Model file for the job. Use its own axes, mm. Face numbers are marked on the shaded views. A direction names the side the tool comes from. Give positions to 0.01 mm unless a question says otherwise; leave off trailing zeros. Order: outer loops, then holes, each group sorted by start corner. A loop starts at its lowest first (then second) coordinate and runs counter-clockwise, first axis right, second up. Notation, with made-up numbers: (-29, 28) -> (-23, 28) arc R28 cw to (-23, 58) -> close; hole circle Ø1 at (-37, 20.5). An arc over 180 degrees is marked (long way). Answer in a Markdown table with one row per item. Add a question column.
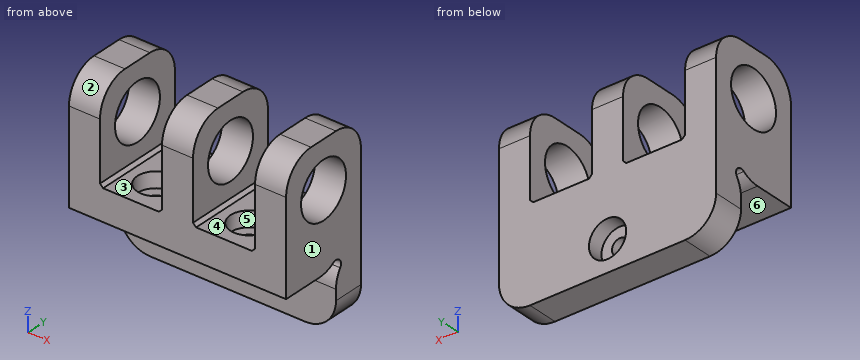
from build123d import *

# Parameters (mm, degrees)
SZKIC1_W                    = 70
SZKIC1_H                    = 30
DODANIE_WYCI_GNI_CIE1_DEPTH = 10
SZKIC2_W                    = 70
SZKIC2_H                    = 10
DODANIE_WYCI_GNI_CIE2_DEPTH = 20
SZKIC3_R                    = 2
WYTNIJ_WYCI_GNI_CIE1_DEPTH  = 75.330343737
ZAOKR_GLENIE1_R             = 10
SZKIC4_W                    = 10
SZKIC4_H                    = 30
DODANIE_WYCI_GNI_CIE3_DEPTH = 30
SZKIC5_R                    = 2.6
WYTNIJ_WYCI_GNI_CIE2_DEPTH  = 49.476798574
SZKIC6_R                    = 6
WYTNIJ_WYCI_GNI_CIE3_DEPTH  = 5
SZKIC7_R                    = 2.6
WYTNIJ_WYCI_GNI_CIE4_DEPTH  = 62.032778079
SZKIC8_R                    = 6
WYTNIJ_WYCI_GNI_CIE5_DEPTH  = 5
ZAOKR_GLENIE2_R             = 10
SZKIC9_R                    = 9
WYTNIJ_WYCI_GNI_CIE6_DEPTH  = 83.006097334
SFAZOWANIE1_SIZE            = 1


with BuildPart() as part:
    # Szkic1 → Dodanie-wyciągnięcie1 (new body)
    with BuildSketch(Plane.XY):
        Rectangle(SZKIC1_W, SZKIC1_H)
    extrude(amount=DODANIE_WYCI_GNI_CIE1_DEPTH)

    # Szkic2 → Dodanie-wyciągnięcie2 (add)
    with BuildSketch(Plane(origin=(0, 0, 0), x_dir=(-1, 0, 0), z_dir=(0, 0, -1))):
        with Locations((0, 10)):
            Rectangle(SZKIC2_W, SZKIC2_H)
    extrude(amount=DODANIE_WYCI_GNI_CIE2_DEPTH)

    # Szkic3 → Wytnij-wyciągnięcie1 (cut, through all)
    with BuildSketch(Plane(origin=(35, 0, 0), x_dir=(0, 0, -1), z_dir=(1, 0, 0))):
        with Locations((0, 5)):
            Circle(SZKIC3_R)
    extrude(amount=-WYTNIJ_WYCI_GNI_CIE1_DEPTH, mode=Mode.SUBTRACT)

    # Zaokrąglenie1
    zaokr_glenie1_edges = [part.edges().sort_by_distance(p)[0] for p in [
        (0, 5, -2),
        (0, 3, 0),
    ]]
    fillet(zaokr_glenie1_edges, radius=ZAOKR_GLENIE1_R)

    # Szkic4 → Dodanie-wyciągnięcie3 (add)
    with BuildSketch(Plane.XY.offset(10)):
        with Locations((-30, 0)):
            Rectangle(SZKIC4_W, SZKIC4_H)
        Rectangle(SZKIC4_W, SZKIC4_H)
        with Locations((30, 0)):
            Rectangle(SZKIC4_W, SZKIC4_H)
    extrude(amount=DODANIE_WYCI_GNI_CIE3_DEPTH)

    # Szkic5 → Wytnij-wyciągnięcie2 (cut, through all)
    with BuildSketch(Plane.XY.offset(10)):
        with Locations((-15, -5)):
            Circle(SZKIC5_R)
    wytnij_wyci_gni_cie2 = extrude(amount=-WYTNIJ_WYCI_GNI_CIE2_DEPTH, mode=Mode.SUBTRACT)

    # Szkic6 → Wytnij-wyciągnięcie3 (cut)
    with BuildSketch(Plane.XY.offset(10)):
        with Locations((-15, -5)):
            Circle(SZKIC6_R)
    wytnij_wyci_gni_cie3 = extrude(amount=-WYTNIJ_WYCI_GNI_CIE3_DEPTH, mode=Mode.SUBTRACT)

    # Lustro1: Wytnij-wyciągnięcie2, Wytnij-wyciągnięcie3 across plane
    add(wytnij_wyci_gni_cie2.mirror(Plane.ZY), mode=Mode.SUBTRACT)
    add(wytnij_wyci_gni_cie3.mirror(Plane.ZY), mode=Mode.SUBTRACT)

    # Szkic7 → Wytnij-wyciągnięcie4 (cut, through all)
    with BuildSketch(Plane(origin=(0, 15, 0), x_dir=(1, 0, 0), z_dir=(0, 1, 0))):
        with Locations(Location((0, 10, 0), (0, 0, 270))):
            Circle(SZKIC7_R)
    extrude(amount=-WYTNIJ_WYCI_GNI_CIE4_DEPTH, mode=Mode.SUBTRACT)

    # Szkic8 → Wytnij-wyciągnięcie5 (cut)
    with BuildSketch(Plane(origin=(0, 15, 0), x_dir=(1, 0, 0), z_dir=(0, 1, 0))):
        with Locations(Location((0, 10, 0), (0, 0, 270))):
            Circle(SZKIC8_R)
    extrude(amount=-WYTNIJ_WYCI_GNI_CIE5_DEPTH, mode=Mode.SUBTRACT)

    # Zaokrąglenie2
    zaokr_glenie2_edges = [part.edges().sort_by_distance(p)[0] for p in [
        (35, 10, -20),
        (-35, 10, -20),
        (-30, -15, 40),
        (-30, 15, 40),
        (0, -15, 40),
        (0, 15, 40),
        (30, 15, 40),
        (30, -15, 40),
    ]]
    fillet(zaokr_glenie2_edges, radius=ZAOKR_GLENIE2_R)

    # Szkic9 → Wytnij-wyciągnięcie6 (cut, through all)
    with BuildSketch(Plane(origin=(35, 0, 0), x_dir=(0, 0, -1), z_dir=(1, 0, 0))):
        with Locations((-25, 0)):
            Circle(SZKIC9_R)
    extrude(amount=-WYTNIJ_WYCI_GNI_CIE6_DEPTH, mode=Mode.SUBTRACT)

    # Sfazowanie1
    sfazowanie1_edges = [part.edges().sort_by_distance(p)[0] for p in [
        (-25, 0, 10),
        (-5, 0, 10),
        (5, 0, 10),
        (25, 0, 10),
    ]]
    chamfer(sfazowanie1_edges, length=SFAZOWANIE1_SIZE)


solid = part.part
Item 1: Which spindle directions (+Z, -Z, +X, -X, +Y, -Y) get a long thin tool onto all of the face, cutting with end or side? Do the marked faces 4, 5 and 6. Say none if no direction does.
Item 2: Saw through at A-A on x = 0. List the corners of the cut face in (y, z), plus the area to 3 significant figures.
Item 3: Saw through at D-D on z = 18. List the corners of the cut face in (x, y).
Item 4: Saw through at C-C on x = 15. List the corners of the cut face in (y, z), plus the area to 3 significant figures.
Item 5: Two-plate mould, pull along X, no slides. Class the marked faces 1, 2 and 3: pulls with the +X half, pulls with the -X half, needs draft (parallel to the pull), parting line crosses it, or undercut.
Item 6: Saw through at B-B on z = 36. List the corners of the cut face in (x, y), plus the area to 3 significant figures.
Item 7: Pin check, flat tips, straight feed: pin 1 Ø6 at (y, z) = (4.5, 27) entering from +X; pin 2 Ø6 at (x, z) = (0, -10) entering from +Y; pin 3 Ø3 at (x, z) = (-12, -8) entering from -Y; pin 4 Ø8.5 at (x, y) = (-15, -5) entering from +Z. Stop position of each tip, or through.
Item 8: Wall check: line 1 (X direction, y = 5, z = 12); line 2 (Y direction, x = 27.5, z = 25); line 3 (Y direction, x = -15, z = 6). Give the ranges that are in metal, low to high.
Evaluation:
| question | item | result |
|---|---|---|
| 1 | face 4 | +Z, +Y, -Y |
| 1 | face 5 | +Z |
| 1 | face 6 | -Z, +X, -X, -Y |
| 2 | outline | (-15, 0) -> (-1.63, 0) arc R10 ccw to (3.89, 1.67) arc R2 cw to (6.67, -1.11) arc R10 ccw to (5, -6.63) -> (5, -7.4) -> (10, -7.4) -> (10, -4) -> (15, -4) -> (15, 30) arc R10 ccw to (5, 40) -> (-5, 40) arc R10 ccw to (-15, 30) -> close; (5, -20) -> (15, -20) -> (15, -16) -> (10, -16) -> (10, -12.6) -> (5, -12.6) -> close; hole circle Ø18 at (0, 25) |
| 2 | area | 1,000 mm2 |
| 3 | outline | (-35, -15) -> (-25, -15) -> (-25, -5.66) -> (-35, -5.66) -> close; (-35, 5.66) -> (-25, 5.66) -> (-25, 15) -> (-35, 15) -> close; (-5, -15) -> (5, -15) -> (5, -5.66) -> (-5, -5.66) -> close; (-5, 5.66) -> (5, 5.66) -> (5, 15) -> (-5, 15) -> close; (25, -15) -> (35, -15) -> (35, -5.66) -> (25, -5.66) -> close; (25, 5.66) -> (35, 5.66) -> (35, 15) -> (25, 15) -> close |
| 4 | outline | (-15, 0) -> (-7.6, 0) -> (-7.6, 5) -> (-11, 5) -> (-11, 10) -> (-15, 10) -> close; (-2.4, 0) -> (-1.63, 0) arc R10 ccw to (3.89, 1.67) arc R2 cw to (6.67, -1.11) arc R10 ccw to (5, -6.63) -> (5, -20) -> (15, -20) -> (15, 10) -> (1, 10) -> (1, 5) -> (-2.4, 5) -> close |
| 4 | area | 401 mm2 |
| 5 | face 1 | pulls with the +X half |
| 5 | face 2 | needs draft |
| 5 | face 3 | undercut |
| 6 | outline | (-35, -13) -> (-25, -13) -> (-25, 13) -> (-35, 13) -> close; (-5, -13) -> (5, -13) -> (5, 13) -> (-5, 13) -> close; (25, -13) -> (35, -13) -> (35, 13) -> (25, 13) -> close |
| 6 | area | 780 mm2 |
| 7 | pin 1 | passes through |
| 7 | pin 2 | stops at y = 10 |
| 7 | pin 3 | stops at y = 5 |
| 7 | pin 4 | stops at z = 5 |
| 8 | line 1 | x = -35 to -25, -5 to 5, 25 to 35 |
| 8 | line 2 | y = -15 to -9, 9 to 15 |
| 8 | line 3 | y = -15 to -11, 1 to 15 |
